Input: part model. Units: mm. Frame: model coordinates. Coordinates: 2 decimals unless noted, no trailing zeros. Order: outer loops, then holes, each group sorted by start corner. A loop starts at its lowest first (then second) coordinate and runs counter-clockwise, first axis right, second up. Notation, with made-up numbers: (-4.5, 66.5) -> (49.5, 66.5) arc R33 cw to (49.5, 104.5) -> close; hole circle Ø5 at (21.5, -32.5). An arc over 180 degrees is marked (long way). Write each question's results on one line, items separated by ' | '.
```python
from build123d import *

# Parameters (mm, degrees)
SKETCH1_R           = 10.25
SKETCH1_R_2         = 4.1
BOSS_EXTRUDE1_DEPTH = 4.05
SKETCH4_R           = 1.25
CUT_EXTRUDE1_DEPTH  = 5.05
CIRPATTERN1_COUNT   = 4
CHAMFER1_SIZE       = 0.4


with BuildPart() as part:
    # Sketch1 → Boss-Extrude1 (new body)
    with BuildSketch(Plane(origin=(0, 0, 0), x_dir=(1, 0, 0), z_dir=(0, 1, 0))):
        Circle(SKETCH1_R)
        Circle(SKETCH1_R_2, mode=Mode.SUBTRACT)
    extrude(amount=-BOSS_EXTRUDE1_DEPTH)

    # Sketch4 → Cut-Extrude1 (cut, through all)
    with BuildSketch(Plane(origin=(0, 0, 0), x_dir=(1, 0, 0), z_dir=(0, 1, 0))):
        with Locations((0, 8)):
            Circle(SKETCH4_R)
    cut_extrude1 = extrude(amount=-CUT_EXTRUDE1_DEPTH, mode=Mode.SUBTRACT)

    # CirPattern1: Cut-Extrude1 ×4 about axis
    cirpattern1_axis = Axis((0, 0, 0), (0, 1, 0))
    for i in range(1, CIRPATTERN1_COUNT):
        add(cut_extrude1.rotate(cirpattern1_axis, i * 360 / CIRPATTERN1_COUNT), mode=Mode.SUBTRACT)

    # Chamfer1
    chamfer1_edges = [part.edges().sort_by_distance(p)[0] for p in [
        (-1.25, -4.05, -8),
        (-1.25, 0, -8),
        (-10.25, 0, 0),
        (-8, -4.05, 1.25),
        (-8, 0, 1.25),
        (1.25, -4.05, 8),
        (1.25, 0, 8),
        (8, -4.05, -1.25),
        (8, 0, -1.25),
        (-10.25, -4.05, 0),
        (-4.1, -4.05, 0),
        (-4.1, 0, 0),
    ]]
    chamfer(chamfer1_edges, length=CHAMFER1_SIZE)


solid = part.part
```
(1) Mould query, pull axis X, two halves, no side actions, for faces 1 (the face through (-2.222, -2.002, 10.006)), 2 (the face through (-6.78, -2, 0.27)), 3 (the face through (2.1, -4.05, 4.2)). Classes: +X half, -X half, draft (parallel to the pull), parting line (faces both ways), or undercut.
Return value:
face 1: parting line | face 2: undercut | face 3: draft
(2) Pin query (flat end, axial travel): P1, Ø1.5, axis at y = -1.5, z = 7, coming from the +X side; P2, Ø8, axis at x = -1, z = 6, coming from the +Y side; P3, Ø3, axis at x = 0, z = -8, coming from the +Y side; P4, Ø3, axis at x = -8, z = 0, coming from the -Y side. Return the tip coordinate at first contact, or that it passes through.
Return value:
P1: x = 8.12 | P2: y = 0 | P3: y = -0.15 | P4: y = -3.9
(3) Line query: line 1 along Z through (x, y) = (0, -2); line 2 along X through (y, z) = (-0.9, -1.5); line 3 along Z through (x, y) = (2, -1.1). Output: solid intervals per line, ascending. Write a range as from..to.
Return value:
line 1: -10.25..-9.25, -6.75..-4.1, 4.1..6.75, 9.25..10.25 | line 2: -10.14..-3.82, 3.82..10.14 | line 3: -10.05..-3.58, 3.58..10.05
(4) Cut plane A-A, the plane x = 0. Count the separate pieces of the cut face and the enclosed holes in it, plus the area to 3 significant figures.
Return value:
separate pieces: 4 | enclosed holes: 0 | area: 28.3 mm2
(5) Cut plane C-C, the plane y = -3.15. Return loops of the section in (x, z), plus the area to 3 significant figures.
Return value:
outline: circle Ø20.5 at (0, 0); hole circle Ø2.5 at (-8, 0); hole circle Ø8.2 at (0, 0); hole circle Ø2.5 at (0, -8); hole circle Ø2.5 at (0, 8); hole circle Ø2.5 at (8, 0) | area: 258 mm2
